Autodesk Inventor part; units mm, degrees
ref_plane "YZ Plane" through (0, 0, 0) normal (1, 0, 0) x (0, 1, 0)
ref_plane "XZ Plane" through (0, 0, 0) normal (0, 1, 0) x (-1, 0, 0)
ref_plane "XY Plane" through (0, 0, 0) normal (0, 0, 1) x (1, 0, 0)
sketch "Sketch1" plane through (0, 0, 0) normal (0, 0, 1) x (1, 0, 0)
  circle A0 centre (0, 0) radius 2.5
  dimension "d0" = 5
extrude "Extrusion1" add sketch "Sketch1" along normal blind 2
fillet "Fillet1" radius 0.5 1 edges at (-2.5, 0, 0)
fillet "Fillet2" radius 1.5 1 edges at (-2.5, 0, 2)
sketch "Sketch2" plane through (0, 0, 2) normal (0, 0, 1) x (1, 0, 0)
  circle A0 centre (0, 0) radius 1
  line L0 (1.75, 0.5) -> (1.75, -0.5)
  line L1 (-1.75, -0.5) -> (-1.75, 0.5)
  line L2 (-0.5, 1.75) -> (0.5, 1.75)
  line L3 (0.5, -1.75) -> (-0.5, -1.75)
  line L4 (-0.5, -1.75) -> (-0.5, -0.5)
  line L5 (-0.5, 0.5) -> (-0.5, 1.75)
  line L6 (-1.75, 0.5) -> (-0.5, 0.5)
  line L7 (0.5, 0.5) -> (1.75, 0.5)
  line L8 (0.5, 1.75) -> (0.5, 0.5)
  line L9 (0.5, -0.5) -> (0.5, -1.75)
  line L10 (1.75, -0.5) -> (0.5, -0.5)
  line L11 (-0.5, -0.5) -> (-1.75, -0.5)
  dimension "d5" = 1
  dimension "d6" = 3.5
  dimension "d7" = 1.75
  dimension "d9" = 1
  dimension "d10" = 3.5
  dimension "d11" = 1.75
extrude "Extrusion2" cut sketch "Sketch2" against normal blind 1.5 contours A0 L10 L9 L4 L11 L6 L5 L8 L7 | A0 L7 L0 L10 | A0 L5 L2 L8 | L9 L3 L4 A0 | A0 L11 L1 L6
chamfer "Chamfer1" distance 1 angle 45 4 edges at (-1.75, 0, 0.5) (0, 1.75, 0.5) (1.75, 0, 0.5) (0, -1.75, 0.5)
chamfer "Chamfer2" distance 0.25 angle 45 4 edges at (-0.5, 0.5, 1.25) (-0.5, -0.5, 1.25) (0.5, 0.5, 1.25) (0.5, -0.5, 1.25)
sketch "Sketch3" plane through (0, 0, 0) normal (0, 0, -1) x (-1, 0, 0)
  circle A0 centre (0, 0) radius 2
  circle A1 centre (0, 0) radius 1.5
  dimension "d19" = 3
extrude "Extrusion3" add sketch "Sketch3" along normal blind 5 contours A1
thread "Thread1"
properties part number "screw_M3_5"
Geometry: final body of the model. Coordinates: model frame, mm. Round coordinates to 2 decimals unless told otherwise and drop trailing zeros. Loops run counter-clockwise (first coordinate to the right, second up) from the corner with the lowest first, then second, coordinate; pieces in that order, holes last. Notation, with made-up numbers: M 37,-26.5 L 71,-26.5 A19 cw 71,-16.5 Z; hole C -35.75,4 d1. An arc over 180 degrees is marked long. Put each result on its own line as item: value. Start each with the question number.
(1) Contact query for flat-ended pins moving along their axis: pin 1 Ø1.5 at (x, z) = (-0.5, -0.5) entering from +Y; pin 2 Ø0.5 at (y, z) = (1.5, 1.5) entering from +X; pin 3 Ø1.1 at (y, z) = (-1.5, 1.5) entering from +X. Output: stop coordinate, or through.
(2) Material intervals for line 1 along Y through (x, z) = (-1.4, 1.75); line 2 along Y through (x, z) = (-0.05, -2); line 3 along X through (y, z) = (0.85, 1), sorted ascending. Write a range as [from, to].
(3) Section query A-A (z = -0.5). Return loops of the section in (x, y), then the cut area to 3 significant figures.
(4) Draft query along Y for faces 1 (the face through (0, 0, -5)), 2 (the face through (0.01, -1.24, 0.99)), 3 (the face through (1.5, -0.07, -2.46)). Return one class per face: +Y half, -Y half, draft (parallel to the pull), parting line (faces both ways), or undercut.
(5) Section query B-B (z = 0.25). Return loops of the section in (x, y), then the cut area to 3 significant figures.
Findings below:
1. pin 1: stops at y = 2.4
1. pin 2: stops at x = 1.83
1. pin 3: stops at x = 2.09
2. line 1: y = [-1.18, -0.5], [0.5, 1.18]
2. line 2: y = [-1.5, 1.5]
2. line 3: x = [-2.26, -0.5], [0.5, 2.26]
3. outline: C 0,0 d3
3. area: 7.07 mm2
4. face 1: draft
4. face 2: undercut
4. face 3: parting line
5. outline: C 0,0 d4.87
5. area: 18.6 mm2
